from build123d import *

# Parameters (mm, degrees)
CROQUIS1_R              = 7.5
CROQUIS1_R_2            = 4
SALIENTE_EXTRUIR1_DEPTH = 30
CROQUIS2_W              = 6.9
CROQUIS2_H              = 3.426383691
SALIENTE_EXTRUIR2_DEPTH = 20
CROQUIS3_R              = 3.925
CORTAR_EXTRUIR1_DEPTH   = 20


with BuildPart() as part:
    # Croquis1 → Saliente-Extruir1 (new body)
    with BuildSketch(Plane(origin=(0, 0, 0), x_dir=(1, 0, 0), z_dir=(0, 1, 0))):
        with Locations(Location((0, 0, 0), (0, 0, 270))):
            Circle(CROQUIS1_R)
        with Locations(Location((0, 0, 0), (0, 0, 270))):
            Circle(CROQUIS1_R_2, mode=Mode.SUBTRACT)
    extrude(amount=SALIENTE_EXTRUIR1_DEPTH)

    # Croquis2 → Saliente-Extruir2 (add)
    with BuildSketch(Plane.XZ):
        with Locations((0, 4.613191846)):
            Rectangle(CROQUIS2_W, CROQUIS2_H)
    extrude(amount=-SALIENTE_EXTRUIR2_DEPTH)

    # Croquis3 → Cortar-Extruir1 (cut)
    with BuildSketch(Plane(origin=(0, 30, 0), x_dir=(1, 0, 0), z_dir=(0, 1, 0))):
        Circle(CROQUIS3_R)
    extrude(amount=-CORTAR_EXTRUIR1_DEPTH, mode=Mode.SUBTRACT)


solid = part.part
Here's how the part is built. I have some questions about the finished solid (model axes, mm). A direction names the side the tool comes from. Coordinates: 2 decimals unless noted, no trailing zeros. Loops run counter-clockwise (first coordinate to the right, second up) from the corner with the lowest first, then second, coordinate; pieces in that order, holes last.
1. Imagine slicing it at C-C, the plane y = 14.25. Please give me the cut outline in (x, z) (3 decimals).
2. For P1, Ø1, axis at y = 4, z = -2, coming from the +X side; P2, Ø3, axis at x = 2, y = 10, coming from the -Z side; P3, Ø3, axis at y = 26.5, z = 5.5, coming from the -X side, each with a flat end and sliding along its axis, tell me the tip position at first contact or that it passes through.
3. Imagine slicing it at A-A, the plane x = 0. Please give me the cut outline in (y, z) (3 decimals), and give its area (3 significant figures).
4. Imagine slicing it at D-D, the plane z = -1.5. Please give me the cut outline in (x, y).
5. Imagine slicing it at B-B, the plane z = 0. Please give me the cut outline in (x, y), and give its area (3 significant figures).
6. If we mould it in two halves opening along X, with no side actions, what happens to faces 1 (the flat face through (0, 10, 3.3)), 2 (the flat face through (-3, 30, 3)), 3 (the cylindrical face through (0.33, 14.79, -7.493))? For each: pulls with the +X half, pulls with the -X half, needs draft (parallel to the pull), parting line crosses it, or undercut.
7. I need wall thicknesses on L1, parallel to X at y = 18.25, z = 0; L2, parallel to X at y = 7.5, z = -1; L3, parallel to Z at x = -3, y = 15.25. Which ranges of each line are inside material? Lowest first, please.
8. For faces 4 (the cylindrical face through (-0.041, 15.07, 3.925)), 5 (the flat face through (0, 5, 2.9)), 6 (the flat face through (0.1, 0, 3.2)), which set-ups out of +Z, -Z, +X, -X, +Y, -Y let a thin tool reach every point of the face, with its end or its side?
Taken from the geometry:
1. outline: circle Ø15 at (0, 0); hole (-2.755, 2.9) arc R4 ccw (long way) to (2.755, 2.9) - (2.645, 2.9) arc R3.925 ccw to (-2.645, 2.9) - close
2. P1: stops at x = 7.35
2. P2: stops at z = -7.48
2. P3: stops at x = -6.34
3. outline: (0, -7.5) - (30, -7.5) - (30, -4) - (0, -4) - close; (0, 2.9) - (10, 2.9) - (10, 3.925) - (20, 3.925) - (20, 4) - (30, 4) - (30, 7.5) - (0, 7.5) - close
3. area: 222 mm2
4. outline: (-7.35, 0) - (-3.71, 0) - (-3.71, 30) - (-7.35, 30) - close; (3.71, 0) - (7.35, 0) - (7.35, 30) - (3.71, 30) - close
5. outline: (-7.5, 0) - (-4, 0) - (-4, 30) - (-7.5, 30) - close; (4, 0) - (7.5, 0) - (7.5, 30) - (4, 30) - close
5. area: 210 mm2
6. face 1: undercut
6. face 2: needs draft
6. face 3: parting line crosses it
7. L1: x = -7.5 to -4, 4 to 7.5
7. L2: x = -7.43 to -3.87, 3.87 to 7.43
7. L3: z = -6.87 to -2.65, 2.65 to 6.87
8. face 4: +Y
8. face 5: +Y, -Y
8. face 6: +Z, -Z, +X, -X, -Y
